Autodesk Inventor part; units mm, degrees
ref_plane "YZ Plane" through (0, 0, 0) normal (1, 0, 0) x (0, 1, 0)
ref_plane "XZ Plane" through (0, 0, 0) normal (0, 1, 0) x (-1, 0, 0)
ref_plane "XY Plane" through (0, 0, 0) normal (0, 0, 1) x (1, 0, 0)
sketch "Sketch1" plane through (0, 0, 0) normal (0, 0, 1) x (1, 0, 0)
  circle A0 centre (0, 0) radius 7.5
  circle A1 centre (0, 0) radius 5.5
  circle A2 centre (0, 0) radius 5
extrude "Extrusion1" add sketch "Sketch1" against normal blind 50 contours A2
sketch "Sketch2" plane through (0, 0, 0) normal (0, 0, 1) x (1, 0, 0)
  point P0 (0, 0)
sketch "Sketch3" plane through (0, 0, 0) normal (0, 0, 1) x (1, 0, 0)
  circle A0 centre (0, 0) radius 5
extrude "Extrusion2" add sketch "Sketch3" along normal blind 150
sketch "Sketch4" plane through (0, 0, 150) normal (0, 0, 1) x (1, 0, 0)
  circle A0 centre (0, 0) radius 5
  circle A1 centre (0, 0) radius 4
  dimension "d4" = 8
extrude "Extrusion3" cut sketch "Sketch4" against normal blind 30
sketch "Sketch5" plane through (0, 0, -50) normal (0, 0, -1) x (-1, 0, 0)
  circle A0 centre (0, 0) radius 5
extrude "Extrusion4" add sketch "Sketch5" along normal blind 20
sketch "Szkic6" plane through (0, 0, -70) normal (0, 0, -1) x (-1, 0, 0)
  circle A0 centre (0, 0) radius 4
  circle A1 centre (0, 0) radius 5
extrude "Wyciągnięcie proste5" add sketch "Szkic6" along normal blind 6 contours A0 | A1
properties part number "os_napedowa"
Source: CAD feature listing. Evaluate the final solid. Frame: model axes, mm. A direction names the side the tool comes from. Round coordinates to 2 decimals unless told otherwise and drop trailing zeros. Order: outer loops, then holes, each group sorted by start corner. A loop starts at its lowest first (then second) coordinate and runs counter-clockwise, first axis right, second up. Notation, with made-up numbers: (58.25, -29.5) -> (84.25, -29.5) arc R11 ccw to (84.25, -21.5) -> close; hole circle Ø6 at (66, 39.5). An arc over 180 degrees is marked (long way). Answer as CSV lines item,"result".
Item 1: Section C-C, the plane z = 125.5. Return loops of the section in (x, y), plus the area to 3 significant figures.
A:
outline,"circle Ø8 at (0, 0)"
area,"50.3 mm²"
Item 2: Pin query (flat end, axial travel): pin 1 Ø3 at (y, z) = (2, -42) entering from +X; pin 2 Ø1 at (y, z) = (-3, 12) entering from -X; pin 3 Ø3 at (x, z) = (4, -8) entering from -Y. Return the tip coordinate at first contact, or that it passes through.
A:
pin 1,"x = 4.97"
pin 2,"x = -4.33"
pin 3,"y = -4.33"
Item 3: Section A-A, the plane x = 0. Return loops of the section in (y, z).
A:
outline,"(-5, -76) -> (5, -76) -> (5, 120) -> (4, 120) -> (4, 150) -> (-4, 150) -> (-4, 120) -> (-5, 120) -> close"
Item 4: Section D-D, the plane z = 2.5. Return loops of the section in (x, y).
A:
outline,"circle Ø10 at (0, 0)"
Item 5: Line query: L1, parallel to Z at x = -3.25, y = 3.75; L2, parallel to X at y = -0.25, z = 107.5; L3, parallel to Y at x = -3, z = 43. Output: solid intervals per line, ascending.
A:
L1,"-76 to 120"
L2,"-4.99 to 4.99"
L3,"-4 to 4"
Item 6: Reachability of faces 1 (the face through (-0.867, -3.905, 135.21)), 2 (the face through (0, 0, -76)) from +Z, -Z, +X, -X, +Y, -Y: full face, straight path, thin tool, end or side. Return the list, or none.
A:
face 1,"+Z"
face 2,"-Z, +X, -X, +Y, -Y"
